Model file for the job. Use its own axes, mm. A direction names the side the tool comes from. Round coordinates to 2 decimals unless told otherwise and drop trailing zeros. Loops run counter-clockwise (first coordinate to the right, second up) from the corner with the lowest first, then second, coordinate; pieces in that order, holes last. Notation, with made-up numbers: (47.5, 21) - (82.5, 21) arc R15 cw to (82.5, 49) - close; hole circle Ø4 at (-5.5, -7.5). An arc over 180 degrees is marked (long way). Answer as a JSON object with one key per item and string values.
from build123d import *

# Parameters (mm, degrees)
SKETCH_R        = 12.5875
PAD_DEPTH       = 10.25
SKETCH005_R     = 17.35
PAD002_DEPTH    = 1.5875
SKETCH004_R     = 11.3
POCKET002_DEPTH = 10.251


with BuildPart() as part:
    # Sketch → Pad (new body)
    with BuildSketch(Plane.XY):
        Circle(SKETCH_R)
    extrude(amount=PAD_DEPTH)

    # Sketch005 (on Face2 of Pad) → Pad002 (new body)
    with BuildSketch(Plane(origin=(0, 0, 0), x_dir=(1, 0, 0), z_dir=(0, 0, -1))):
        Circle(SKETCH005_R)
    extrude(amount=-PAD002_DEPTH)

    # Sketch004 (on Face3 of Pad) → Pocket002 (cut, through all)
    with BuildSketch(Plane.XY.offset(10.25)):
        Circle(SKETCH004_R)
    extrude(amount=-POCKET002_DEPTH, mode=Mode.SUBTRACT)


solid = part.part
1) Tool access for faces 1 (the flat face through (11, 4, 0)), 2 (the flat face through (-9.1, -9.1, 1.588)): list every direction of +Z, -Z, +X, -X, +Y, -Y with a clear straight run to the whole face (end or side of a thin tool).
Values follow:
{"face 1": "-Z, +X, -X, +Y, -Y", "face 2": "+Z"}
2) Slice it at D-D on x = -14. List the corners of the cut face in (y, z), then the cut area to 3 significant figures.
Values follow:
{"outline": "(-10.25, 0) - (10.25, 0) - (10.25, 1.59) - (-10.25, 1.59) - close", "area": "32.5 mm²"}
3) Slice it at A-A on y = 0. List the corners of the cut face in (x, z).
Values follow:
{"outline": "(-17.35, 0) - (-11.3, 0) - (-11.3, 10.25) - (-12.59, 10.25) - (-12.59, 1.59) - (-17.35, 1.59) - close; (11.3, 0) - (17.35, 0) - (17.35, 1.59) - (12.59, 1.59) - (12.59, 10.25) - (11.3, 10.25) - close"}
4) Probe probe 1 along Y at (x, z) = (0, 7.5); probe 2 along Z at (x, y) = (11, 12.5); probe 3 along X at (y, z) = (-1, 3.5). List the from-to ranges inside material, lowest first.
Values follow:
{"probe 1": "-12.59 to -11.3, 11.3 to 12.59", "probe 2": "0 to 1.59", "probe 3": "-12.55 to -11.26, 11.26 to 12.55"}
5) Slice it at C-C on z = 8.25. List the corners of the cut face in (x, y) (1 decimal), then the cut area to 3 significant figures.
Values follow:
{"outline": "circle Ø25.2 at (0, 0); hole circle Ø22.6 at (0, 0)", "area": "96.6 mm²"}
6) Two-plate mould, pull along X, no slides. Class faces 3 (the cylindrical face through (10.78, 3.39, 5.2)), 4 (the flat face through (-9.4, 6.6, 10.25)), 5 (the cylindrical face through (-2.259, -17.202, 0.783)): pulls with the +X half, pulls with the -X half, needs draft (parallel to the pull), parting line crosses it, or undercut.
Values follow:
{"face 3": "undercut", "face 4": "needs draft", "face 5": "parting line crosses it"}
7) Drop flat-ended pins along their axis: P1, Ø4, axis at x = -13, z = 2, coming from the -Y side; P2, Ø4, axis at x = -12.5, z = 4.5, coming from the +Y side; P3, Ø4, axis at y = 12, z = 7, coming from the -X side; P4, Ø12, axis at x = 2.5, y = 2, coming from the -Z side. Give the stop position or say it passes through.
Values follow:
{"P1": "y = -13.38", "P2": "y = 6.94", "P3": "x = -7.64", "P4": "through"}
